Geometry check sheet. Reference: the model listing, model coordinates, mm. Face numbers are marked on the shaded views. A direction names the side the tool comes from. Round coordinates to 2 decimals unless told otherwise and drop trailing zeros. Order: outer loops, then holes, each group sorted by start corner. A loop starts at its lowest first (then second) coordinate and runs counter-clockwise, first axis right, second up. Notation, with made-up numbers: M 44.5,79 L 72.5,79 A27 ccw 72.5,118 Z; hole C -16.75,38 d11. An arc over 180 degrees is marked long. Answer as a JSON object with one key per item and string values. Group by question number.
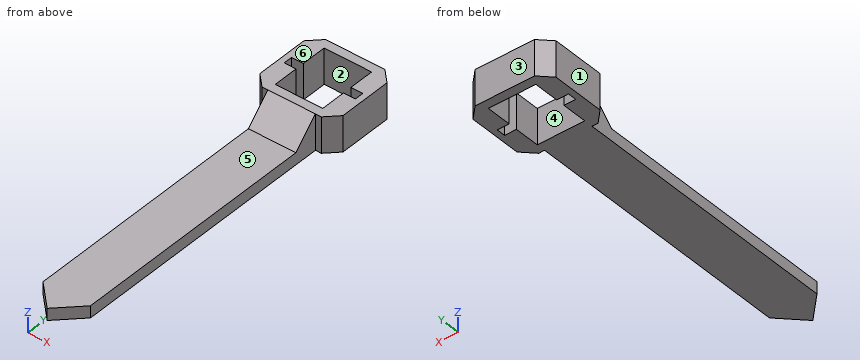
```python
from build123d import *

# Parameters (mm, degrees)
F1_DEPTH = 6
F0_W     = 8
F0_H     = 50
F2_DEPTH = 2
F3_SIZE  = 3.99999
F4_SIZE  = 2


# Not quite as in the source:
# - a fillet or chamfer is up to 0.001 mm smaller than in the source, because OpenCascade refuses the exact size


with BuildPart() as f1:
    # F0 (on Top) → F1 (new body)
    with BuildSketch(Plane.XY):
        Polygon((4, -6.5), (7, -6.5), (7, 6.5), (-7, 6.5), (-7, -6.5), (-4, -6.5), align=None)
        Polygon((4, -0.75), (4, -5), (-4, -5), (-4, -0.75), (-6, -0.75), (-6, 0.75), (-4, 0.75), (-4, 5), (4, 5), (4, 0.75), (6, 0.75), (6, -0.75), align=None, mode=Mode.SUBTRACT)
    extrude(amount=F1_DEPTH)

    # F0 (on Top) → F2 (join)
    with BuildSketch(Plane.XY):
        with Locations((0, -31.5)):
            Rectangle(F0_W, F0_H)
    extrude(amount=F2_DEPTH)

    # F3 (size 4 in the source; OpenCascade refuses exactly that, so slightly less here)
    f3_edges = [f1.edges().sort_by_distance(p)[0] for p in [
        (0, -6.5, 2),
        (-4, -56.5, 1),
        (4, -56.5, 1),
    ]]
    chamfer(f3_edges, length=F3_SIZE)

    # F4
    f4_edges = [f1.edges().sort_by_distance(p)[0] for p in [
        (-7, -6.5, 3),
        (-7, 6.5, 3),
        (7, -6.5, 3),
        (7, 6.5, 3),
    ]]
    chamfer(f4_edges, length=F4_SIZE)


solid = f1.part
```
1) Sectioned sample at A-A (y = 1.5). Record the boundary of the cut face in (x, z), then the cut area to 3 significant figures.
2) Set-up check for the marked faces 4, 5 and 6: record each of +Z, -Z, +X, -X, +Y, -Y from which the full face is reachable in a straight line by a thin tool's end or side.
3) Thickness scan on line 1 along Y through (x, z) = (4.75, 3.55); line 2 along X through (y, z) = (1, 2.5); line 3 along X through (y, z) = (0.5, 0.8). Record the ranges inside material, lowest first. Write a range as [from, to].
4) Go/stop test with flat-tipped pins: P1, Ø8, axis at x = -4.5, y = -39.5, coming from the +Z side; P2, Ø3, axis at y = -45.5, z = 2, coming from the +X side; P3, Ø0.6, axis at x = -5, z = 2, coming from the -Y side; P4, Ø1.8, axis at y = -18.5, z = 4, coming from the +X side. Record where each tip stops, or that it passes through.
5) Release check for a two-part mould opening along X. For the marked faces 1, 2 and 3 record: +X half, -X half, draft (parallel to the pull), parting line (faces both ways), or undercut.
Final values:
{
 "1": {"outline": "M -7,0 L -4,0 L -4,6 L -7,6 Z; M 4,0 L 7,0 L 7,6 L 4,6 Z", "area": "36.0 mm^2"},
 "2": {"face 4": "+Z, -Z", "face 5": "+Z, +X, -X, -Y", "face 6": "+Z, +X, -X, +Y, -Y"},
 "3": {"line 1": "y = [-6.5, -0.75], [0.75, 6.5]", "line 2": "x = [-7, -4], [4, 7]", "line 3": "x = [-7, -6], [6, 7]"},
 "4": {"P1": "stops at z = 2", "P2": "stops at x = 4", "P3": "stops at y = -6.5", "P4": "passes through"},
 "5": {"face 1": "-X half", "face 2": "undercut", "face 3": "draft"}
}
